Design review of the part built by this model. Coordinates are the model's own, in mm. Face numbers are marked on the shaded views. Give positions to 0.01 mm unless a question says otherwise; leave off trailing zeros. Write each loop counter-clockwise with the first axis right and the second up, starting at its lowest first coordinate (ties: lowest second). Pieces come first, ordered by that corner, then holes. Notation, with made-up numbers: (40, 70) -> (99, 70) arc R16 ccw to (99, 78) -> close; hole circle Ø2 at (-25.5, 84.25). An arc over 180 degrees is marked (long way). Write each question's results on one line, items separated by ' | '. Start each with the question number.
(1) Take a section at B-B (x = 1). State the section outline as (y, z) points, plus the area to 3 significant figures.
(2) Take a section at C-C (y = 3.75). State the section outline as (x, z) points.
(3) Take a section at D-D (z = -7.25). State the section outline as (x, y) points.
(4) Mouldability with a two-part tool opening along X and no side actions: class the marked faces 1, 2 and 3 as released by +X, released by -X, zero draft, split by the parting line, or undercut.
(5) Clearance check with flat-ended pins moving along their axes: pin 1 (3 mm diameter, centred on x = -1, z = 1, fed in from -Y); pin 2 (2 mm diameter, centred on y = 3, z = -7.5, fed in from +X); pin 3 (2 mm diameter, centred on x = 5, z = 5.5, fed in from -Y); pin 4 (1.5 mm diameter, centred on x = 8.5, y = 6, fed in from +Z). State where each tip first meets the part, or that it passes through.
(6) To check wall thickness, follow probe 1 along X at (y, z) = (0.15, 0); probe 2 along X at (y, z) = (4, 0). State the ranges of each line that lie inside material, in increasing order.
(7) Take a section at A-A (z = 0). State the section outline as (x, y) points, plus the area to 3 significant figures.
Autodesk Inventor part; units mm, degrees
ref_plane "YZ Plane" through (0, 0, 0) normal (1, 0, 0) x (0, 1, 0)
ref_plane "XZ Plane" through (0, 0, 0) normal (0, 1, 0) x (-1, 0, 0)
ref_plane "XY Plane" through (0, 0, 0) normal (0, 0, 1) x (1, 0, 0)
sketch "Sketch1" plane through (0, 0, 0) normal (1, 0, 0) x (0, 1, 0)
  line L0 (0, 0) -> (7, 0) construction
  line L1 (7, 0) -> (7, -4) construction
  line L2 (7, -4) -> (0, -4)
  line L3 (0, -4) -> (0, 0) construction
  line L4 (7, -11) -> (0, -11)
  line L5 (7, -5) -> (6.8, -5)
  line L6 (6.8, -5) -> (6.8, -10)
  line L7 (6.8, -10) -> (7, -10)
  line L8 (0, -5) -> (0.2, -5)
  line L9 (0.2, -5) -> (0.2, -10)
  line L10 (0.2, -10) -> (0, -10)
  line L11 (7, -4) -> (7, -5)
  line L12 (7, -10) -> (7, -11)
  line L13 (0, -11) -> (0, -10)
  line L14 (0, -5) -> (0, -4)
  dimension "d0" = 4
  dimension "d2" = 7
  dimension "d5" = 11
  dimension "d6" = 0.2
  dimension "d7" = 1
revolve "Revolution1" add sketch "Sketch1" angle 360 about axis through (0, 0, 0) along (0, 1, 0)
properties part number "608 bearing"
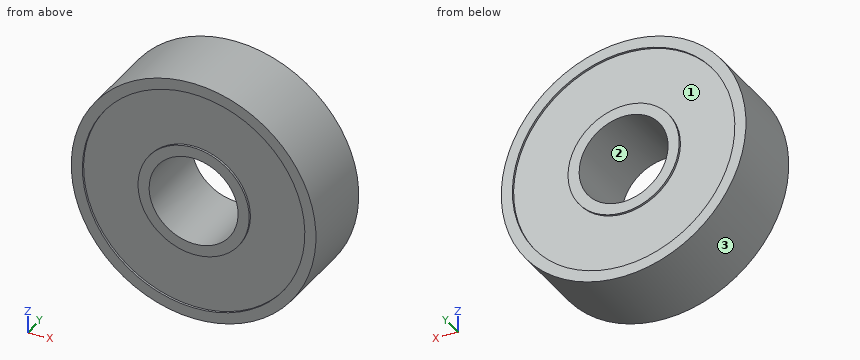
Report:
1) outline: (0, -10.95) -> (7, -10.95) -> (7, -9.95) -> (6.8, -9.95) -> (6.8, -4.9) -> (7, -4.9) -> (7, -3.87) -> (0, -3.87) -> (0, -4.9) -> (0.2, -4.9) -> (0.2, -9.95) -> (0, -9.95) -> close; (0, 3.87) -> (7, 3.87) -> (7, 4.9) -> (6.8, 4.9) -> (6.8, 9.95) -> (7, 9.95) -> (7, 10.95) -> (0, 10.95) -> (0, 9.95) -> (0.2, 9.95) -> (0.2, 4.9) -> (0, 4.9) -> close | area: 95.1 mm2
2) outline: circle Ø22 at (0, 0); hole circle Ø8 at (0, 0)
3) outline: (-8.27, 0) -> (-6.89, 0) -> (-6.89, 0.2) -> (6.89, 0.2) -> (6.89, 0) -> (8.27, 0) -> (8.27, 7) -> (6.89, 7) -> (6.89, 6.8) -> (-6.89, 6.8) -> (-6.89, 7) -> (-8.27, 7) -> close
4) face 1: undercut | face 2: undercut | face 3: split by the parting line
5) pin 1: through | pin 2: x = 8.87 | pin 3: y = 0.2 | pin 4: z = 7.81
6) probe 1: -11 to -10, -5 to -4, 4 to 5, 10 to 11 | probe 2: -11 to -4, 4 to 11
7) outline: (-11, 0) -> (-10, 0) -> (-10, 0.2) -> (-5, 0.2) -> (-5, 0) -> (-4, 0) -> (-4, 7) -> (-5, 7) -> (-5, 6.8) -> (-10, 6.8) -> (-10, 7) -> (-11, 7) -> close; (4, 0) -> (5, 0) -> (5, 0.2) -> (10, 0.2) -> (10, 0) -> (11, 0) -> (11, 7) -> (10, 7) -> (10, 6.8) -> (5, 6.8) -> (5, 7) -> (4, 7) -> close | area: 94.0 mm2
